Check sheet for the drawn part. Datum: minimum x, y, z corner. Units: mm. Give positions to 0.01 mm unless a question says otherwise; leave off trailing zeros. Write each loop counter-clockwise with the first axis right and the second up, starting at its lowest first coordinate (ties: lowest second). Pieces come first, ordered by that corner, then holes. Notation, with made-up numbers: (-31.75, 40.25) -> (22.25, 40.25) arc R34 ccw to (22.25, 72.25) -> close; hole circle Ø11 at (44.5, 18). An arc over 180 degrees is marked (long way). Use CSV: the item, a comma, the result in double quotes. Start each with the question number.
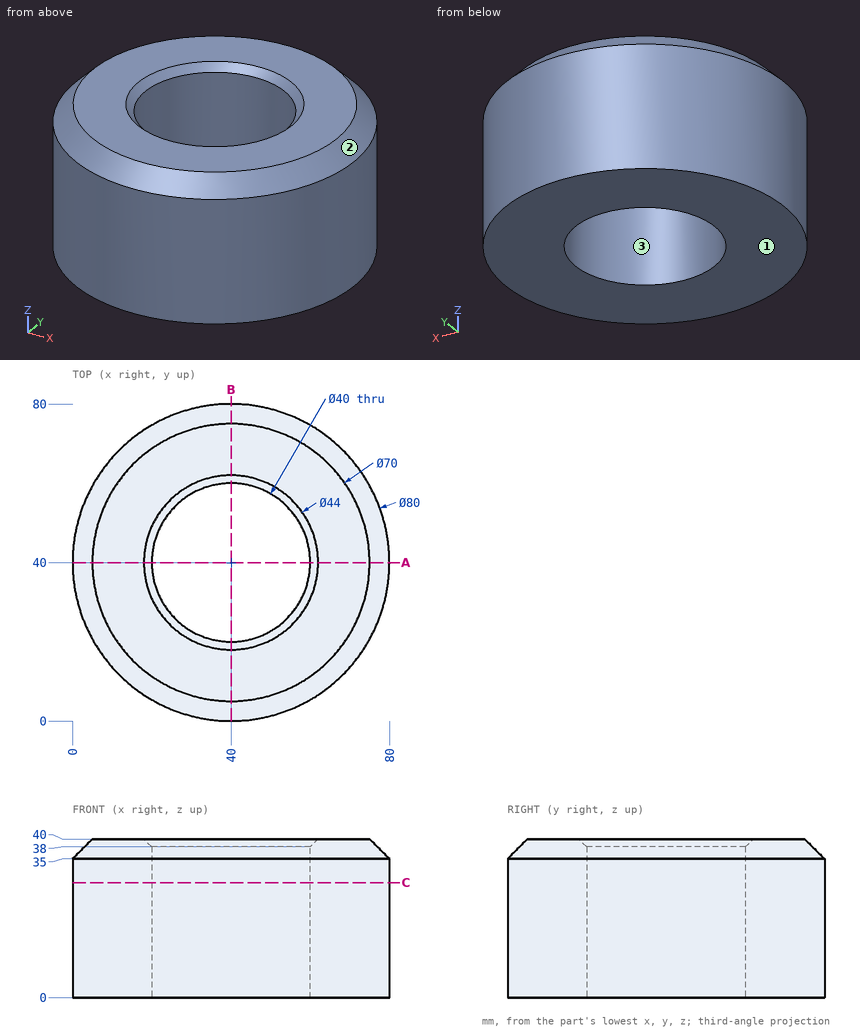
(1) Go/stop test with flat-tipped pins: pin 1 (5 mm diameter, centred on y = 17, z = 17, fed in from +X); pin 2 (3 mm diameter, centred on x = 12.5, y = 66, fed in from +Z); pin 3 (3 mm diameter, centred on x = 10.5, y = 52.5, fed in from -Z); pin 4 (1 mm diameter, centred on y = 55.5, z = 16.5, fed in from -X). Record where each tip stops, or that it passes through.
(2) Thickness scan on line 1 (Y direction, x = 40, z = 8); line 2 (Y direction, x = 22.5, z = 4); line 3 (X direction, y = 27, z = 37). Record the ranges inside material, lowest first. Write a range as from..to.
(3) Draft check along Y on the marked faces 1, 2 and 3. Enter one of: released by +Y, released by -Y, zero draft, split by the parting line, or undercut.
(4) Section check A-A on y = 40. Record the cut outline in (x, z).
(5) Section check C-C on z = 29. Record the cut outline in (x, y), then the cut area to 3 significant figures.
Data:
1,pin 1,"stops at x = 74.35"
1,pin 2,"stops at z = 38.65"
1,pin 3,"stops at z = 0"
1,pin 4,"stops at x = 2.92"
2,line 1,"y = 0..20, 60..80"
2,line 2,"y = 4.03..30.32, 49.68..75.97"
2,line 3,"x = 4.29..24.8, 55.2..75.71"
3,face 1,"zero draft"
3,face 2,"split by the parting line"
3,face 3,"undercut"
4,outline,"(0, 0) -> (20, 0) -> (20, 38) -> (18, 40) -> (5, 40) -> (0, 35) -> close; (60, 0) -> (80, 0) -> (80, 35) -> (75, 40) -> (62, 40) -> (60, 38) -> close"
5,outline,"circle Ø80 at (40, 40); hole circle Ø40 at (40, 40)"
5,area,"3,770 mm2"
